Geometry check sheet. Reference: the model listing, model coordinates, mm. A direction names the side the tool comes from. Round coordinates to 2 decimals unless told otherwise and drop trailing zeros. Loops run counter-clockwise (first coordinate to the right, second up) from the corner with the lowest first, then second, coordinate; pieces in that order, holes last. Notation, with made-up numbers: (-36.75, 57.5) -> (-2.75, 57.5) arc R26 cw to (-2.75, 71.5) -> close; hole circle Ø7 at (-18.75, -29.5). An arc over 180 degrees is marked (long way). Use a Markdown table: item, result. Add a question column.
Q1. Gauge pin test, flat ends, axial feed: P1, Ø1.5, axis at x = -1, z = 26.5, coming from the -Y side; P2, Ø0.7, axis at x = 0.5, z = 68, coming from the -Y side. Record the tip position at first contact, or that the pin passes through.
Q2. Material ranges on L1, parallel to Z at x = 0.35, y = 1.35; L2, parallel to Y at x = 1, z = 32.5, recorded low to high.
Q3. Sectioned sample at A-A, the plane x = 0. Enter the section's corners in (y, z), then the cut area to 3 significant figures.
Q4. Release check for a two-part mould opening along X. For faces 4 (the face through (0, 0, 70)), 5 (the face through (-1.5, 0.07, 34.51)) record: released by +X, released by -X, zero draft, split by the parting line, or undercut.
Q5. Sectioned sample at B-B, the plane z = 14.5. Enter the section's corners in (x, y), then the cut area to 3 significant figures.
Q6. Set-up check for faces 1 (the face through (0, 0, 0)), 2 (the face through (0, 1, 68)), 3 (the face through (0, -1, 68)): record each of +Z, -Z, +X, -X, +Y, -Y from which the full face is reachable in a straight line by a thin tool's end or side.
```python
from build123d import *

# Parameters (mm, degrees)
SKETCH_1_R          = 1.5
EXTRUDE_1_DEPTH     = 70
SKETCH_2_W          = 4
SKETCH_2_H          = 1
CUT_EXTRUDE_2_DEPTH = 4


with BuildPart() as part:
    # 草图1 → 凸台-拉伸1 (new body)
    with BuildSketch(Plane.XY):
        Circle(SKETCH_1_R)
    extrude(amount=EXTRUDE_1_DEPTH)

    # 草图2 → 切除-拉伸2 (cut)
    with BuildSketch(Plane.XY.offset(70)):
        with Locations((0.214520216, -1.5)):
            Rectangle(SKETCH_2_W, SKETCH_2_H)
        with Locations((0.214520216, 1.5)):
            Rectangle(SKETCH_2_W, SKETCH_2_H)
    extrude(amount=-CUT_EXTRUDE_2_DEPTH, mode=Mode.SUBTRACT)


solid = part.part
```
Values:
| question | item | result |
|---|---|---|
| 1 | P1 | y = -1.48 |
| 1 | P2 | y = -1 |
| 2 | L1 | 0 to 66 |
| 2 | L2 | -1.12 to 1.12 |
| 3 | outline | (-1.5, 0) -> (1.5, 0) -> (1.5, 66) -> (1, 66) -> (1, 70) -> (-1, 70) -> (-1, 66) -> (-1.5, 66) -> close |
| 3 | area | 206 mm^2 |
| 4 | face 4 | zero draft |
| 4 | face 5 | split by the parting line |
| 5 | outline | circle Ø3 at (0, 0) |
| 5 | area | 7.07 mm^2 |
| 6 | face 1 | -Z, +X, -X, +Y, -Y |
| 6 | face 2 | +Z, +X, -X, +Y |
| 6 | face 3 | +Z, +X, -X, -Y |
